Geometry check sheet. Reference: the model listing, model coordinates, mm. Face numbers are marked on the shaded views. A direction names the side the tool comes from. Round coordinates to 2 decimals unless told otherwise and drop trailing zeros. Loops run counter-clockwise (first coordinate to the right, second up) from the corner with the lowest first, then second, coordinate; pieces in that order, holes last.
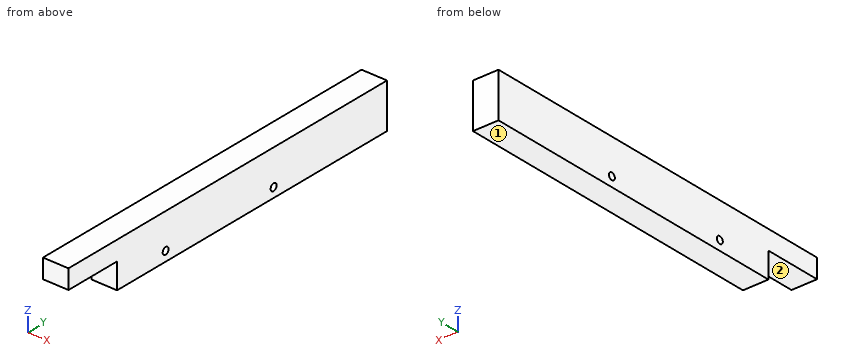
```python
from build123d import *

# Parameters (mm, degrees)
F0_W     = 40
F0_H     = 70
F1_DEPTH = 500
F3_D     = 11
F3_DEPTH = 50
F4_W     = 40
F4_H     = 30
F5_DEPTH = 90


with BuildPart() as f1:
    # F0 (on Front) → F1 (new body)
    with BuildSketch(Plane.XZ):
        with Locations((20, 35)):
            Rectangle(F0_W, F0_H)
    extrude(amount=F1_DEPTH)

    # F3
    with Locations(Plane.YZ.offset(40)):
        with Locations((-410, 15), (-210, 15)):
            Hole(F3_D / 2, depth=F3_DEPTH)

    # F4 (on face) → F5 (join)
    with BuildSketch(Plane.XZ.offset(500)):
        with Locations((20, 55)):
            Rectangle(F4_W, F4_H)
    extrude(amount=F5_DEPTH)


solid = f1.part
```
1) Gauge pin test, flat end, axial feed: pin 1 (6.5 mm diameter, centred on y = -210, z = 15, fed in from -X). Record the tip position at first contact, or that the pin passes through.
Report:
pin 1: passes through
2) Sectioned sample at A-A, the plane x = 32.5. Record the cut outline in (y, z).
Report:
outline: (-590, 40) - (-500, 40) - (-500, 0) - (0, 0) - (0, 70) - (-590, 70) - close; hole circle Ø11 at (-410, 15); hole circle Ø11 at (-210, 15)
3) Scan lines: line 1 along Z through (x, y) = (31, -410); line 2 along Y through (x, z) = (16, 12.5); line 3 along Y through (x, z) = (29.5, 23.5). Record each from-to range of solid material in increasing order.
Report:
line 1: z = 0 to 9.5, 20.5 to 70
line 2: y = -500 to -414.9, -405.1 to -214.9, -205.1 to 0
line 3: y = -500 to 0
4) Sectioned sample at B-B, the plane y = -410. Record the cut outline in (x, z).
Report:
outline: (0, 0) - (40, 0) - (40, 9.5) - (0, 9.5) - close; (0, 20.5) - (40, 20.5) - (40, 70) - (0, 70) - close
5) Access from +Z, -Z, +X, -X, +Y, -Y to the whole of each face (thin tool, end or side, straight path). Record for the marked faces 1 and 2.
Report:
face 1: -Z, +X, -X, +Y, -Y
face 2: -Z, +X, -X, -Y
